Autodesk Inventor part; units mm, degrees
ref_plane "YZ Plane" through (0, 0, 0) normal (1, 0, 0) x (0, 1, 0)
ref_plane "XZ Plane" through (0, 0, 0) normal (0, 1, 0) x (-1, 0, 0)
ref_plane "XY Plane" through (0, 0, 0) normal (0, 0, 1) x (1, 0, 0)
sketch "Sketch1" plane through (0, 0, 0) normal (0, 0, 1) x (1, 0, 0)
  line L0 (-505, 165) -> (443.2, 165)
  line L1 (443.2, 165) -> (443.2, -165)
  line L2 (443.2, -165) -> (-505, -165)
  line L3 (-505, -165) -> (-505, 165)
  line L4 (0, 231) -> (0, -231)
  line L5 (-694.64, 0) -> (632.84, 0)
  line L6 (3.2, 108.4) -> (18, 108.4)
  line L7 (18, 108.4) -> (18, -108.4)
  line L8 (18, -108.4) -> (3.2, -108.4)
  line L9 (3.2, -108.4) -> (3.2, 108.4)
  line L10 (-101.8, 108.4) -> (-87, 108.4)
  line L11 (-87, 108.4) -> (-87, -108.4)
  line L12 (-87, -108.4) -> (-101.8, -108.4)
  line L13 (-101.8, -108.4) -> (-101.8, 108.4)
  line L14 (-206.8, 108.4) -> (-192, 108.4)
  line L15 (-192, 108.4) -> (-192, -108.4)
  line L16 (-192, -108.4) -> (-206.8, -108.4)
  line L17 (-206.8, -108.4) -> (-206.8, 108.4)
  line L18 (-311.8, 108.4) -> (-297, 108.4)
  line L19 (-297, 108.4) -> (-297, -108.4)
  line L20 (-297, -108.4) -> (-311.8, -108.4)
  line L21 (-311.8, -108.4) -> (-311.8, 108.4)
  line L22 (-416.8, 108.4) -> (-402, 108.4)
  line L23 (-402, 108.4) -> (-402, -108.4)
  line L24 (-402, -108.4) -> (-416.8, -108.4)
  line L25 (-416.8, -108.4) -> (-416.8, 108.4)
  line L26 (108.2, 108.4) -> (123, 108.4)
  line L27 (123, 108.4) -> (123, -108.4)
  line L28 (123, -108.4) -> (108.2, -108.4)
  line L29 (108.2, -108.4) -> (108.2, 108.4)
  line L30 (213.2, 108.4) -> (228, 108.4)
  line L31 (228, 108.4) -> (228, -108.4)
  line L32 (228, -108.4) -> (213.2, -108.4)
  line L33 (213.2, -108.4) -> (213.2, 108.4)
  line L34 (318.2, 108.4) -> (333, 108.4)
  line L35 (333, 108.4) -> (333, -108.4)
  line L36 (333, -108.4) -> (318.2, -108.4)
  line L37 (318.2, -108.4) -> (318.2, 108.4)
  line L38 (438, 108.4) -> (423.2, 108.4)
  line L39 (423.2, 108.4) -> (423.2, -108.4)
  line L40 (423.2, -108.4) -> (438, -108.4)
  line L41 (438, -108.4) -> (438, 108.4)
  line L42 (-505, 159) -> (443.2, 159) construction
  line L43 (-505, -159) -> (443.2, -159) construction
  circle A0 centre (-416.1, 159) radius 3
  circle A1 centre (-190.1, 159) radius 3
  circle A2 centre (35.9, 159) radius 3
  circle A3 centre (261.9, 159) radius 3
  circle A4 centre (-460.3, 159) radius 3
  circle A5 centre (-416.1, -159) radius 3
  circle A6 centre (-190.1, -159) radius 3
  circle A7 centre (261.9, -159) radius 3
  circle A8 centre (-460.3, -159) radius 3
  circle A9 centre (35.9, -159) radius 3
  point P0 (0, 0)
  dimension "d1" = 330
  dimension "d2" = 216.8
  dimension "d3" = 14.8
  dimension "d5" = 14.8
  dimension "d8" = 14.8
  dimension "d9" = 14.8
  dimension "d11" = 14.8
  dimension "d14" = 14.8
  dimension "d16" = 14.8
  dimension "d18" = 14.8
  dimension "d20" = 438
  dimension "d21" = 14.8
  dimension "d24" = 105
  dimension "d25" = 105
  dimension "d26" = 105
  dimension "d27" = 105
  dimension "d28" = 105
  dimension "d29" = 105
  dimension "d30" = 105
  dimension "d31" = 105
  dimension "d32" = 505
  dimension "d33" = 5.2
  dimension "d34" = 6
  dimension "d35" = 6
  dimension "d36" = 6
  dimension "d37" = 88.9
  dimension "d38" = 88.9
  dimension "d39" = 226
  dimension "d40" = 226
  dimension "d41" = 226
  dimension "d42" = 226
  dimension "d43" = 226
  dimension "d44" = 226
  dimension "d45" = 44.7
  dimension "d46" = 44.7
extrude "Extrusion1" add sketch "Sketch1" along normal blind 5 contours L0 L4 L5 L11 L10 L13 L15 L14 L17 L19 L18 L21 L23 L22 L25 L3 | L0 L1 L5 L41 L38 L39 L35 L34 L37 L31 L30 L33 L27 L26 L29 L7 L6 L9 L4 | L5 L25 L24 L23 L21 L20 L19 L17 L16 L15 L13 L12 L11 L4 L2 L3 | L5 L9 L8 L7 L29 L28 L27 L33 L32 L31 L37 L36 L35 L39 L40 L41 L1 L2 L4
properties part number "FerriteLayer"
The listing builds one solid part. Answer for the finished solid, in the listing's coordinates (mm). Give positions to 0.01 mm unless a question says otherwise; leave off trailing zeros.
Item 1: This flat-tipped pin is pushed along its axis until it touches: pin 1 Ø1.5 at (x, y) = (109.5, 17) entering from -Z. Where does it stop, or does it pass through?
Derived:
pin 1: passes through
Item 2: Find the intervals of material crossed by line 1 along X through (y, z) = (159, 2.75); line 2 along Y through (x, z) = (261.9, 3.9); line 3 along Y through (x, z) = (-416.1, 1.8), in increasing order.
Derived:
line 1: x = -505 to -463.3, -457.3 to -419.1, -413.1 to -193.1, -187.1 to 32.9, 38.9 to 258.9, 264.9 to 443.2
line 2: y = -165 to -162, -156 to 156, 162 to 165
line 3: y = -165 to -162, -156 to -108.4, 108.4 to 156, 162 to 165
Item 3: A cutting plane is placed at A-A (y = 48.5). Give the number of separate pieces and of enclosed holes in the cut face, then the cut area to 4 significant figures.
Derived:
separate pieces: 10
enclosed holes: 0
area: 4,075 mm2
